```python
from build123d import *

# Parameters (mm, degrees)
BOSS_EXTRUDE1_DEPTH = 4
SKETCH2_R           = 1
BOSS_EXTRUDE2_DEPTH = 3.5
SKETCH3_W           = 5
SKETCH3_H           = 10
BOSS_EXTRUDE3_DEPTH = 10
SKETCH4_R           = 1.55
CUT_EXTRUDE1_DEPTH  = 3
SKETCH4_3_R         = 1.55
CUT_EXTRUDE2_DEPTH  = 5
SKETCH7_R           = 3
CUT_EXTRUDE3_DEPTH  = 2
SKETCH8_R           = 1
CUT_EXTRUDE4_DEPTH  = 2
SKETCH9_R           = 1
CUT_EXTRUDE5_DEPTH  = 2
CUT_EXTRUDE6_DEPTH  = 4
SKETCH6_R           = 1.55
CUT_EXTRUDE7_DEPTH  = 3
SKETCH6_3_R         = 1.55
CUT_EXTRUDE8_DEPTH  = 5


with BuildPart() as part:
    # Sketch1 → Boss-Extrude1 (new body)
    with BuildSketch(Plane(origin=(0, 0, 0), x_dir=(1, 0, 0), z_dir=(0, 1, 0))):
        with BuildLine():
            Line((0, 80), (0, 0))
            Line((0, 0), (126, 0))
            ThreePointArc((126, 0), (128.828427125, 1.171572875), (130, 4))
            Line((130, 4), (130, 76))
            ThreePointArc((130, 76), (128.828427125, 78.828427125), (126, 80))
            Line((126, 80), (0, 80))
        make_face()
    extrude(amount=BOSS_EXTRUDE1_DEPTH)

    # Sketch2 → Boss-Extrude2 (add)
    with BuildSketch(Plane(origin=(0, 0, 0), x_dir=(-1, 0, 0), z_dir=(0, -1, 0))):
        with Locations(Location((-125.5, 4.5, 0), (0, 0, 270))):
            Circle(SKETCH2_R)
        with Locations(Location((-125.5, 75.5, 0), (0, 0, 270))):
            Circle(SKETCH2_R)
    extrude(amount=BOSS_EXTRUDE2_DEPTH)

    # Sketch3 → Boss-Extrude3 (add)
    with BuildSketch(Plane(origin=(0, 0, 0), x_dir=(-1, 0, 0), z_dir=(0, -1, 0))):
        with Locations((-14.5, 7.2)):
            Rectangle(SKETCH3_W, SKETCH3_H)
        with Locations((-14.5, 72.8)):
            Rectangle(SKETCH3_W, SKETCH3_H)
    extrude(amount=BOSS_EXTRUDE3_DEPTH)

    # Sketch4 → Cut-Extrude1 (cut)
    with BuildSketch(Plane(origin=(17, 0, 0), x_dir=(0, 0, -1), z_dir=(1, 0, 0))):
        Polygon((3.535898385, -4.923428426), (5.201636264, -7.961714213), (8.665737879, -8.038285787), (10.464101615, -5.076571574), (8.798363736, -2.038285787), (5.334262121, -1.961714213), align=None)
        with Locations((7, -5)):
            Circle(SKETCH4_R, mode=Mode.SUBTRACT)
    extrude(amount=-CUT_EXTRUDE1_DEPTH, mode=Mode.SUBTRACT)

    # Sketch4<3> → Cut-Extrude2 (cut)
    with BuildSketch(Plane(origin=(17, 0, 0), x_dir=(0, 0, -1), z_dir=(1, 0, 0))):
        with Locations((7, -5)):
            Circle(SKETCH4_3_R)
    extrude(amount=-CUT_EXTRUDE2_DEPTH, mode=Mode.SUBTRACT)

    # Sketch7 → Cut-Extrude3 (cut)
    with BuildSketch(Plane.XZ):
        with Locations(Location((70, -25, 0), (0, 0, 270))):
            Circle(SKETCH7_R)
        with Locations(Location((70, -55, 0), (0, 0, 270))):
            Circle(SKETCH7_R)
    extrude(amount=-CUT_EXTRUDE3_DEPTH, mode=Mode.SUBTRACT)

    # Sketch8 → Cut-Extrude4 (cut)
    with BuildSketch(Plane(origin=(0, 2, 0), x_dir=(-1, 0, 0), z_dir=(0, -1, 0))):
        with Locations(Location((-70, 55, 0), (0, 0, 90))):
            Circle(SKETCH8_R)
    extrude(amount=-CUT_EXTRUDE4_DEPTH, mode=Mode.SUBTRACT)

    # Sketch9 → Cut-Extrude5 (cut)
    with BuildSketch(Plane(origin=(0, 2, 0), x_dir=(-1, 0, 0), z_dir=(0, -1, 0))):
        with Locations(Location((-70, 25, 0), (0, 0, 90))):
            Circle(SKETCH9_R)
    extrude(amount=-CUT_EXTRUDE5_DEPTH, mode=Mode.SUBTRACT)

    # Sketch10 → Cut-Extrude6 (cut)
    with BuildSketch(Plane(origin=(0, 0, 0), x_dir=(-1, 0, 0), z_dir=(0, -1, 0))):
        Polygon((-78, 30), (-40, 30), (-40, 50), (-78, 50), (-78, 65), (-113, 65), (-113, 15), (-78, 15), align=None)
    extrude(amount=-CUT_EXTRUDE6_DEPTH, mode=Mode.SUBTRACT)

    # Sketch6 → Cut-Extrude7 (cut)
    with BuildSketch(Plane(origin=(17, 0, 0), x_dir=(0, 0, -1), z_dir=(1, 0, 0))):
        Polygon((76.464101615, -5), (74.732050808, -2), (71.267949192, -2), (69.535898385, -5), (71.267949192, -8), (74.732050808, -8), align=None)
        with Locations((73, -5)):
            Circle(SKETCH6_R, mode=Mode.SUBTRACT)
    extrude(amount=-CUT_EXTRUDE7_DEPTH, mode=Mode.SUBTRACT)

    # Sketch6<3> → Cut-Extrude8 (cut)
    with BuildSketch(Plane(origin=(17, 0, 0), x_dir=(0, 0, -1), z_dir=(1, 0, 0))):
        with Locations((73, -5)):
            Circle(SKETCH6_3_R)
    extrude(amount=-CUT_EXTRUDE8_DEPTH, mode=Mode.SUBTRACT)


solid = part.part
```
Geometry check sheet. Reference: the model listing, model coordinates, mm. A direction names the side the tool comes from. Round coordinates to 2 decimals unless told otherwise and drop trailing zeros. Order: outer loops, then holes, each group sorted by start corner. A loop starts at its lowest first (then second) coordinate and runs counter-clockwise, first axis right, second up. Notation, with made-up numbers: (34.5, 59.5) -> (64.5, 59.5) arc R21 cw to (64.5, 75.5) -> close; hole circle Ø5 at (-25.5, 67). An arc over 180 degrees is marked (long way). Return JSON: item names as keys, results as strings. Group by question number.
Q1. Section check C-C, the plane z = -7. Record the boundary of the cut face in (x, y).
Q2. Gauge pin test, flat ends, axial feed: pin 1 (6.5 mm diameter, centred on y = -4.5, z = -6.5, fed in from +X); pin 2 (4 mm diameter, centred on x = 14.5, y = -6, fed in from -Z); pin 3 (2.5 mm diameter, centred on x = 13.5, y = -3, fed in from +Z). Record the tip position at first contact, or that the pin passes through.
Q3. Section check A-A, the plane x = 55. Record the boundary of the cut face in (y, z).
Q4. Section check B-B, the plane z = -36. Record the boundary of the cut face in (x, y).
Q5. Material ranges on probe 1 along X at (y, z) = (3.35, -25); probe 2 along X at (y, z) = (1.05, -25); probe 3 along Y at (x, z) = (13.6, -73), recorded low to high. Write a range as from..to.
Q6. Tool access check on faces 1 (the cylindrical face through (68.2, 1, -52.6)), 2 (the flat face through (15.5, -6.5, -75.6)), 3 (the flat face through (15, -5, -67.8)), 4 (the flat face through (59, 2, -50)). Record the directions out of +Z, -Z, +X, -X, +Y, -Y that give a thin tool (end or side, any length) a straight path to the whole face; none if there is none.
Q7. Release check for a two-part mould opening along Z. For faces 5 (the flat face through (62, 2, 0)), 6 (the cylindrical face through (67.07, 0.99, -24.35)), 7 (the flat face through (12, -3.82, -8.24)) record: released by +Z, released by -Z, zero draft, split by the parting line, or undercut.
Numbers:
{
 "1": {"outline": "(0, 0) -> (12, 0) -> (12, -3.45) -> (14, -3.45) -> (14, -2) -> (17, -2) -> (17, 0) -> (130, 0) -> (130, 4) -> (0, 4) -> close; (12, -10) -> (17, -10) -> (17, -8) -> (14, -8) -> (14, -6.55) -> (12, -6.55) -> close"},
 "2": {"pin 1": "x = 126.5", "pin 2": "z = -77.8", "pin 3": "z = -2.2"},
 "3": {"outline": "(0, -80) -> (4, -80) -> (4, -50) -> (0, -50) -> close; (0, -30) -> (4, -30) -> (4, 0) -> (0, 0) -> close"},
 "4": {"outline": "(0, 0) -> (40, 0) -> (40, 4) -> (0, 4) -> close; (113, 0) -> (130, 0) -> (130, 4) -> (113, 4) -> close"},
 "5": {"probe 1": "0..69, 71..78, 113..130", "probe 2": "0..67, 73..78, 113..130", "probe 3": "-10..-6.55, -3.45..4"},
 "6": {"face 1": "-Y", "face 2": "+X", "face 3": "+X, -X, -Y", "face 4": "+Y, -Y"},
 "7": {"face 5": "released by +Z", "face 6": "undercut", "face 7": "zero draft"}
}
